from build123d import *

# Parameters (mm, degrees)
F1_DEPTH = 15.875
F2_R     = 12.7
F3_R     = 76.2


with BuildPart() as f1:
    # F0 (on Right) → F1 (new body)
    with BuildSketch(Plane.YZ):
        Polygon((-355.6, 0), (0, 0), (0, 501.232803), (-229.74942, 521.333272), (-238.604443, 420.119891), (-150.418242, 412.404598), (-178.476583, 91.696291), (-355.6, 76.2), align=None)
    extrude(amount=F1_DEPTH)

    # F2
    f2_edges = [f1.edges().sort_by_distance(p)[0] for p in [
        (7.9375, -355.6, 0),
        (7.9375, 0, 0),
        (7.9375, 0, 501.232803),
        (7.9375, -238.604443, 420.119891),
        (7.9375, -229.74942, 521.333272),
    ]]
    fillet(f2_edges, radius=F2_R)

    # F3
    f3_edges = [f1.edges().sort_by_distance(p)[0] for p in [
        (7.9375, -150.418242, 412.404598),
    ]]
    fillet(f3_edges, radius=F3_R)


solid = f1.part
Design review of the part built by this model. Coordinates are the model's own, in mm. A direction names the side the tool comes from. Coordinates: 2 decimals unless noted, no trailing zeros. Write each loop counter-clockwise with the first axis right and the second up, starting at its lowest first coordinate (ties: lowest second). Pieces come first, ordered by that corner, then holes. Notation, with made-up numbers: (-24, 48.25) -> (31, 48.25) arc R23 ccw to (31, 60.25) -> close; hole circle Ø10 at (24, 1.25). An arc over 180 degrees is marked (long way). Write each question's results on one line, items separated by ' | '. Start each with the question number.
(1) The part is to be moulded in two halves that separate along Z. For faces 3 (the face through (8.049, -226.261, 517.393)), 4 (the face through (7.83, -167.62, 215.81)), 5 (the face through (8.05, -234.68, 423.63)), 6 (the face through (0, -101, 264)), say which applies: pulls with the +Z half, pulls with the -Z half, needs draft (parallel to the pull), parting line crosses it, or undercut.
(2) For line 1 along Y through (x, z) = (9.5, 191.5); line 2 along Z through (x, y) = (9.5, -247); line 3 along Z through (x, y) = (2, -99), list the stretches that pass through material, from the lowest coordinate up. Write a range as from..to.
(3) Tool access review of faces 1 (the face through (7.826, -265.798, 84.057)), 2 (the face through (8, -355.6, 45)): name each direction out of +Z, -Z, +X, -X, +Y, -Y from which nothing blocks a thin tool from reaching the whole face with its end or side.
(4) Take a section at B-B on z = 213. Write out the cut boundary in (x, y) (3 decimals).
(5) Take a section at A-A on y = -277. Write out the cut boundary in (x, z) (3 decimals), and give its area (3 significant figures).
(6) Clearance check with a flat-ended pin moving along its axis: P1, Ø4, axis at x = 7, y = -126.5, coming from the +Z side. State where the tip first meets the part, or that it passes through.
Results found:
1) face 3: pulls with the +Z half | face 4: undercut | face 5: undercut | face 6: needs draft
2) line 1: y = -169.74..0 | line 2: z = 0..85.7 | line 3: z = 0..509.89
3) face 1: +X, -X, -Y | face 2: +Z, -Z, +X, -X, -Y
4) outline: (0, -167.864) -> (15.875, -167.864) -> (15.875, 0) -> (0, 0) -> close
5) outline: (0, 0) -> (15.875, 0) -> (15.875, 83.077) -> (0, 83.077) -> close | area: 1,320 mm2
6) P1: stops at z = 512.48
